from build123d import *

# Parameters (mm, degrees)
SKETCH1_W = 30
SKETCH1_H = 2.5
FILLET1_R = 0.5
FILLET2_R = 1


with BuildPart() as part:
    # Sketch1 → Revolve1 (revolve)
    with BuildSketch(Plane.YZ, mode=Mode.PRIVATE) as revolve1_sk:
        with BuildLine():
            ThreePointArc((-1, 7.5), (-3.222184013, 4.038873605), (-4, 0))
            Line((-4, 0), (0, 0))
            Line((0, 0), (0, 7.5))
            Line((0, 7.5), (-1, 7.5))
        make_face()
        with Locations((15, 1.25)):
            Rectangle(SKETCH1_W, SKETCH1_H)
    revolve(revolve1_sk.sketch.rotate(Axis((0, -13.848615749, 0), (0, 1, 0)), 180), axis=Axis((0, -13.848615749, 0), (0, 1, 0)))

    # Fillet1
    fillet1_edges = [part.edges().sort_by_distance(p)[0] for p in [
        (0, 0, 7.5),
    ]]
    fillet(fillet1_edges, radius=FILLET1_R)

    # Fillet2
    fillet2_edges = [part.edges().sort_by_distance(p)[0] for p in [
        (0, -1, 7.5),
    ]]
    fillet(fillet2_edges, radius=FILLET2_R)


solid = part.part
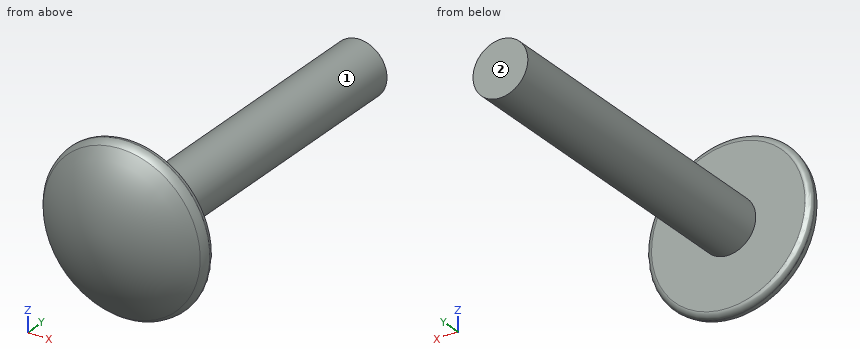
Here's how the part is built. I have some questions about the finished solid (model axes, mm). Face numbers are marked on the shaded views. A direction names the side the tool comes from. Coordinates: 2 decimals unless noted, no trailing zeros. Write each loop counter-clockwise with the first axis right and the second up, starting at its lowest first coordinate (ties: lowest second). Pieces come first, ordered by that corner, then holes.
Item 1: If I drill on line 1 (Y direction, x = -5.25, z = -2); line 2 (Y direction, x = -2.5, z = -4); line 3 (Z direction, x = -1, y = 20), over which ranges is the centre line in solid material (lowest first)?
Item 2: On a 3-axis mill with a long thin cutter (end or side, diameter ignored), from which of +Z, -Z, +X, -X, +Y, -Y can I reach the whole of each face in a straight line? I mean the marked faces 1 and 2. Say none if no direction works.
Item 3: Will these pins go through, and if not, where does the flat tip stop? pin 1 (2 mm diameter, centred on x = -0.5, y = 26, fed in from -Z); pin 2 (2 mm diameter, centred on x = 2, z = 4, fed in from +Y); pin 3 (1.5 mm diameter, centred on y = 6, z = 0, fed in from +X).
Item 4: I want a section at A-A on y = 14. Write out the boundary of the cut face in (x, z).
Findings below:
1. line 1: y = -2.44 to 0
1. line 2: y = -2.92 to 0
1. line 3: z = -2.29 to 2.29
2. face 1: +Y
2. face 2: +Z, -Z, +X, -X, +Y
3. pin 1: stops at z = -2.5
3. pin 2: stops at y = 0
3. pin 3: stops at x = 2.5
4. outline: circle Ø5 at (0, 0)
